from build123d import *

# Parameters (mm, degrees)
SKETCH1_W                = 64
SKETCH1_H                = 17
BOSS_EXTRUDE1_DEPTH      = 12.5
SKETCH2_R                = 6
CUT_EXTRUDE1_DEPTH       = 8
BOSS_EXTRUDE2_DEPTH      = 3
BOSS_EXTRUDE2_DEPTH_BACK = 12.5
SKETCH3_W                = 19
SKETCH3_H                = 44
BOSS_EXTRUDE3_DEPTH      = 19
BOSS_EXTRUDE4_DEPTH      = 57.437921
FILLET2_R                = 0.5
FILLET3_R                = 3


with BuildPart() as part:
    # Sketch1 → Boss-Extrude1 (new body)
    with BuildSketch(Plane(origin=(0, 0, 0), x_dir=(1, 0, 0), z_dir=(0, 1, 0))):
        Polygon((0, 39), (-88, 39), (-98, 29), (-98, 10), (-88, 0), (0, 0), align=None)
        with Locations((-51, 19.5)):
            Rectangle(SKETCH1_W, SKETCH1_H, mode=Mode.SUBTRACT)
    extrude(amount=BOSS_EXTRUDE1_DEPTH)

    # Sketch2 → Cut-Extrude1 (cut)
    with BuildSketch(Plane(origin=(-83, 0, 0), x_dir=(0, 0, -1), z_dir=(1, 0, 0))):
        with Locations((19.5, 6.25)):
            Circle(SKETCH2_R)
    extrude(amount=-CUT_EXTRUDE1_DEPTH, mode=Mode.SUBTRACT)

    # Sketch3 → Boss-Extrude2 (add, two sides: drawn at the far end of the back side and taken through both)
    with BuildSketch(Plane(origin=(0, 12.5, 0), x_dir=(1, 0, 0), z_dir=(0, 1, 0)).offset(-BOSS_EXTRUDE2_DEPTH_BACK)):
        with Locations((-9.5, 19.5)):
            Rectangle(SKETCH3_W, SKETCH3_H)
    extrude(amount=BOSS_EXTRUDE2_DEPTH + BOSS_EXTRUDE2_DEPTH_BACK)

    # Sketch4 → Boss-Extrude3 (add)
    with BuildSketch(Plane(origin=(0, 0, 0), x_dir=(0, 0, -1), z_dir=(1, 0, 0))):
        Polygon((41.5, 15.5), (41.5, 52.420383772), (-2.5, 15.5), align=None)
    extrude(amount=-BOSS_EXTRUDE3_DEPTH)

    # Sketch5 → Boss-Extrude4 (add)
    with BuildSketch(Plane(origin=(0, 52.420383772, -41.5), x_dir=(1, 0, 0), z_dir=(0, -0.6427876096865353, 0.7660444431189817))):
        Polygon((0, 0), (0, 15), (-8, 15), (-6.5, 12), (-5, 12), (-5, 0), align=None)
    extrude(amount=BOSS_EXTRUDE4_DEPTH)

    # Fillet2
    fillet2_edges = [part.edges().sort_by_distance(p)[0] for p in [
        (-5, 33.960191799, -19.499999897),
        (-5, 43.152725117, -11.786548581),
    ]]
    fillet(fillet2_edges, radius=FILLET2_R)

    # Fillet3
    fillet3_edges = [part.edges().sort_by_distance(p)[0] for p in [
        (-4, 63.911050419, -31.858185855),
        (0, 45.450858446, -9.858185752),
        (-4, 26.990666474, 12.141814352),
        (0, 21.24533315, 7.320907279),
        (0, 58.165717095, -36.679092927),
    ]]
    fillet(fillet3_edges, radius=FILLET3_R - 0.0001)  # a hair under: the kernel refuses the full size


solid = part.part
Geometry check sheet. Reference: the model listing, model coordinates, mm. A direction names the side the tool comes from. Round coordinates to 2 decimals unless told otherwise and drop trailing zeros. Loops run counter-clockwise (first coordinate to the right, second up) from the corner with the lowest first, then second, coordinate; pieces in that order, holes last. Notation, with made-up numbers: (-5, -4.5) - (49, -4.5) arc R22 cw to (49, 9.5) - close; hole circle Ø5 at (-25.5, 30). An arc over 180 degrees is marked (long way). One line per question, with ' | ' between items. Start each with the question number.
1. Tool access check on faces 1 (the face through (-86.944, 11.309, -22.726)), 2 (the face through (-5.15, 42.785, -11.57)), 3 (the face through (-59.1, 12.5, -28.4)), 4 (the face through (-54, 6, 0)). Record the directions out of +Z, -Z, +X, -X, +Y, -Y that give a thin tool (end or side, any length) a straight path to the whole face; none if there is none.
2. Scan lines: line 1 (Y direction, x = -86, z = -19.5); line 2 (Z direction, x = -86, y = 6); line 3 (Z direction, x = -21, y = 12). Record each from-to range of solid material in increasing order. Write a range as [from, to].
3. Cross-section at A-A on y = 6.25. Record the cut outline in (x, z), then the cut area to 3 significant figures.
4. Draft check along X on faces 5 (the face through (-6.007, 43.411, -12.095)), 6 (the face through (-0.9, 56.51, -36.95)), 7 (the face through (-51, 6, -11)). Enter one of: released by +X, released by -X, zero draft, split by the parting line, or undercut.
5. Depth check by flat-ended pin: pin 1 (3 mm diameter, centred on x = -31, z = -9, fed in from +Y); pin 2 (6 mm diameter, centred on y = 24, z = -30, fed in from -X); pin 3 (6 mm diameter, centred on x = -44, y = 5.5, fed in from -Z). Enter the tip coordinate at first touch or a pass-through.
6. Cross-section at B-B on x = -34.5. Record the cut outline in (y, z), then the cut area to 3 significant figures.
Taken from the geometry:
1) face 1: none | face 2: -X | face 3: +Z, -Z, -X, +Y | face 4: +Z, -X, +Y, -Y
2) line 1: [0, 0.25], [12.25, 12.5] | line 2: [-39, -25.49], [-13.51, 0] | line 3: [-39, -28], [-11, 0]
3) outline: (-98, -29) - (-88, -39) - (-19, -39) - (-19, -41.5) - (0, -41.5) - (0, 2.5) - (-19, 2.5) - (-19, 0) - (-88, 0) - (-98, -10) - close; hole (-91, -25.5) - (-83, -25.5) - (-83, -28) - (-19, -28) - (-19, -11) - (-83, -11) - (-83, -13.5) - (-91, -13.5) - close | area: 2,630 mm²
4) face 5: zero draft | face 6: released by +X | face 7: undercut
5) pin 1: y = 12.5 | pin 2: x = -19 | pin 3: z = -39
6) outline: (0, -39) - (12.5, -39) - (12.5, -28) - (0, -28) - close; (0, -11) - (12.5, -11) - (12.5, 0) - (0, 0) - close | area: 275 mm²
